Verification items for the finished model (mm, model axes). Round coordinates to 2 decimals unless told otherwise and drop trailing zeros. Loops run counter-clockwise (first coordinate to the right, second up) from the corner with the lowest first, then second, coordinate; pieces in that order, holes last.
from build123d import *

# Parameters (mm, degrees)
SKETCH1_W                       = 39.116
SKETCH1_H                       = 39.116
BOSS_EXTRUDE1_DEPTH             = 12.7
F_21_0_159_DIAMETER_HOLE1_D     = 4.0386
F_21_0_159_DIAMETER_HOLE1_DEPTH = 12.7
F_1_4_0_25_DIAMETER_HOLE1_D     = 6.35
F_1_4_0_25_DIAMETER_HOLE1_DEPTH = 12.7
LPATTERN1_COUNT                 = 2
LPATTERN1_PITCH                 = 12.7
LPATTERN1_COL_COUNT             = 2
LPATTERN1_COL_PITCH             = 12.7
F_1_4_20_TAPPED_HOLE1_D         = 5.1054
F_1_4_20_TAPPED_HOLE1_DEPTH     = 12.7


with BuildPart() as part:
    # Sketch1 → Boss-Extrude1 (new body)
    with BuildSketch(Plane(origin=(0, 0, 0), x_dir=(1, 0, 0), z_dir=(0, 1, 0))):
        Rectangle(SKETCH1_W, SKETCH1_H)
    extrude(amount=BOSS_EXTRUDE1_DEPTH)

    # #21 (0.159) Diameter Hole1
    with Locations(Plane(origin=(0, 12.7, 0), x_dir=(1, 0, 0), z_dir=(0, 1, 0))):
        with Locations((-14.89, 15.928), (-15.398, -16.028), (16.058, -16.028), (16.058, 15.928)):
            Hole(F_21_0_159_DIAMETER_HOLE1_D / 2, depth=F_21_0_159_DIAMETER_HOLE1_DEPTH)

    # 1/4 (0.25) Diameter Hole1
    with Locations(Plane(origin=(0, 12.7, 0), x_dir=(1, 0, 0), z_dir=(0, 1, 0))):
        with Locations((0, 0)):
            f_1_4_0_25_diameter_hole1 = Hole(F_1_4_0_25_DIAMETER_HOLE1_D / 2, depth=F_1_4_0_25_DIAMETER_HOLE1_DEPTH)

    # LPattern1: 1/4 (0.25) Diameter Hole1 ×2
    with Locations(*[(-i * LPATTERN1_PITCH, 0, 0) for i in range(1, LPATTERN1_COUNT)]):
        add(f_1_4_0_25_diameter_hole1, mode=Mode.SUBTRACT)

    # LPattern1 col: 1/4 (0.25) Diameter Hole1 ×2
    with Locations(*[(i * LPATTERN1_COL_PITCH, 0, 0) for i in range(1, LPATTERN1_COL_COUNT)]):
        add(f_1_4_0_25_diameter_hole1, mode=Mode.SUBTRACT)

    # 1/4-20 Tapped Hole1
    with Locations(Plane(origin=(0, 12.7, 0), x_dir=(1, 0, 0), z_dir=(0, 1, 0))):
        with Locations((0, 12.7), (0, -12.690681966)):
            Hole(F_1_4_20_TAPPED_HOLE1_D / 2, depth=F_1_4_20_TAPPED_HOLE1_DEPTH)


solid = part.part
1. Release check for a two-part mould opening along Z. For faces 1 (the face through (0, 6, 19.558)), 2 (the face through (14.972, 6.261, 14.325)), 3 (the face through (-5, 0, 0)) record: released by +Z, released by -Z, zero draft, split by the parting line, or undercut.
2. Section check B-B (x = -14.89). Enter the section's corners in (y, z), then the cut area to 3 significant figures.
3. Section check C-C (y = 1.25). Give the number of separate pieces and of enclosed holes in the cut face, then the cut area to 3 significant figures.
4. Section check A-A (x = 12.7). Enter the section's corners in (y, z) (3 decimals).
5. Gauge pin test, flat end, axial feed: P1, Ø5.5, axis at x = -15.398, z = 16.028, coming from the +Y side. Record the tip position at first contact, or that the pin passes through.
6. Section check D-D (x = -10). Enter the section's corners in (y, z).
7. Scan lines: L1, parallel to Z at x = 0, y = 8 (3 decimals); L2, parallel to X at y = 5, z = 0.5; L3, parallel to X at y = 4.5, z = -12.7. Record each from-to range of solid material in increasing order.
Taken from the geometry:
1. face 1: released by +Z
1. face 2: undercut
1. face 3: zero draft
2. outline: (0, -19.56) - (12.7, -19.56) - (12.7, -17.95) - (0, -17.95) - close; (0, -13.91) - (12.7, -13.91) - (12.7, -2.3) - (0, -2.3) - close; (0, 2.3) - (12.7, 2.3) - (12.7, 14.07) - (0, 14.07) - close; (0, 17.98) - (12.7, 17.98) - (12.7, 19.56) - (0, 19.56) - close
2. area: 337 mm2
3. separate pieces: 1
3. enclosed holes: 9
3. area: 1,340 mm2
4. outline: (0, -19.558) - (12.7, -19.558) - (12.7, -3.175) - (0, -3.175) - close; (0, 3.175) - (12.7, 3.175) - (12.7, 19.558) - (0, 19.558) - close
5. P1: stops at y = 12.7
6. outline: (0, -19.56) - (12.7, -19.56) - (12.7, -1.67) - (0, -1.67) - close; (0, 1.67) - (12.7, 1.67) - (12.7, 19.56) - (0, 19.56) - close
7. L1: z = -19.558 to -15.253, -10.147 to -3.175, 3.175 to 10.138, 15.243 to 19.558
7. L2: x = -19.56 to -15.84, -9.56 to -3.14, 3.14 to 9.56, 15.84 to 19.56
7. L3: x = -19.56 to -2.55, 2.55 to 19.56
